Model file for the job. Use its own axes, mm. A direction names the side the tool comes from. Coordinates: 2 decimals unless noted, no trailing zeros. Write each loop counter-clockwise with the first axis right and the second up, starting at its lowest first coordinate (ties: lowest second). Pieces come first, ordered by that corner, then holes. Notation, with made-up numbers: (75.25, -30.75) - (80.25, -30.75) arc R20 cw to (80.25, -0.75) - close; hole circle Ø11 at (14.25, -14.5). An arc over 180 degrees is marked (long way). Put each result on its own line as item: value. Start each with the question number.
1. Saw through at B-B, the plane y = 68. Give the number of separate pieces and of enclosed holes in the cut face, plus the area to 3 significant figures.
2. Saw through at A-A, the plane x = -1. Write the cut outline in (y, z), plus the area to 3 significant figures.
3. Saw through at D-D, the plane z = 2. Write the cut outline in (x, y), plus the area to 3 significant figures.
4. Which spindle directions (+Z, -Z, +X, -X, +Y, -Y) get a long thin tool onto all of the face, cutting with end or side? Do faces 1 (the face through (102, 41, 76.483)), 2 (the face through (-3, 10, 11.5)), 3 (the face through (102, 31, 115.138)). Say none if no direction does.
5. Drill centre lines: L1, parallel to Y at x = 164.5, z = 72; L2, parallel to Y at x = 167, z = 89; L3, parallel to Z at x = 10, y = 12. Where is each one in solid material? Low to high. Write a range as from..to.
6. Drop flat-ended pins along their axis: P1, Ø16.5, axis at x = 91, z = 2.5, coming from the +Y side; P2, Ø1, axis at x = 7, y = 36.5, coming from the -Z side. Give the stop position or say it passes through.
7. Pull direction Z, two halves, no side cores. Call faces 4 (the face through (203, 15, 0)), 5 (the face through (102, 44.52, 79)), 6 (the face through (108, 5, 0)), 7 (the face through (102, 55, 86.614)): released by +Z, released by -Z, zero draft, split by the parting line, or undercut.
8. Saw through at C-C, the plane y = 8. Write the cut outline in (x, z).
```python
from build123d import *

# Parameters (mm, degrees)
SKETCH_1_W            = 100
SKETCH_1_H            = 50
EXTRUDE_1_DEPTH       = 200
SKETCH_2_W            = 192
SKETCH_2_H            = 92
CUT_EXTRUDE_1_DEPTH   = 20
SKETCH_3_W            = 100
SKETCH_3_H            = 50
EXTRUDE_2_DEPTH       = 20
SKETCH_4_W            = 100
SKETCH_4_H            = 50
EXTRUDE_3_DEPTH       = 20
SKETCH_6_W            = 23
SKETCH_6_H            = 10
CUT_EXTRUDE_2_DEPTH   = 15
SKETCH_7_W            = 23
SKETCH_7_H            = 10
CUT_EXTRUDE_3_DEPTH   = 15
SKETCH_10_R           = 21.643075995
SKETCH_10_R_2         = 21.043075995
SKETCH_10_W           = 0.6
SKETCH_10_H           = 92
CUT_EXTRUDE_2_2_DEPTH = 0.05
EXTRUDE_4_DEPTH       = 240
SKETCH_12_W           = 30.390175899
SKETCH_12_H           = 33.741429703
EXTRUDE_5_DEPTH       = 4
SKETCH_13_W           = 30.390175899
SKETCH_13_H           = 33.741429703
EXTRUDE_6_DEPTH       = 4
SKETCH_14_R           = 0.75
EXTRUDE_7_DEPTH       = 27.291157


with BuildPart() as part:
    # 草圖1 → 填料-伸長1 (new body)
    with BuildSketch(Plane(origin=(0, 0, 0), x_dir=(0, 0, -1), z_dir=(1, 0, 0))):
        Rectangle(SKETCH_1_W, SKETCH_1_H)
    extrude(amount=EXTRUDE_1_DEPTH)

    # 草圖2 → 除料-伸長1 (cut)
    with BuildSketch(Plane(origin=(0, 25, 0), x_dir=(1, 0, 0), z_dir=(0, 1, 0))):
        with Locations((100, 0)):
            Rectangle(SKETCH_2_W, SKETCH_2_H)
    extrude(amount=-CUT_EXTRUDE_1_DEPTH, mode=Mode.SUBTRACT)

    # 草圖3 → 填料-伸長2 (add)
    with BuildSketch(Plane.ZY):
        Rectangle(SKETCH_3_W, SKETCH_3_H)
    extrude(amount=EXTRUDE_2_DEPTH)

    # 草圖4 → 填料-伸長3 (add)
    with BuildSketch(Plane(origin=(200, 0, 0), x_dir=(0, 0, -1), z_dir=(1, 0, 0))):
        Rectangle(SKETCH_4_W, SKETCH_4_H)
    extrude(amount=EXTRUDE_3_DEPTH)

    # 草圖6 → Cut-Extrude 2 (cut)
    with BuildSketch(Plane(origin=(4, 0, 0), x_dir=(0, 0, -1), z_dir=(1, 0, 0))):
        with Locations((0, 10)):
            Rectangle(SKETCH_6_W, SKETCH_6_H)
    extrude(amount=-CUT_EXTRUDE_2_DEPTH, mode=Mode.SUBTRACT)

    # 草圖7 → 除料-伸長3 (cut)
    with BuildSketch(Plane.ZY.offset(-196)):
        with Locations((0, 10)):
            Rectangle(SKETCH_7_W, SKETCH_7_H)
    extrude(amount=-CUT_EXTRUDE_3_DEPTH, mode=Mode.SUBTRACT)

    # 草圖10 → Cut-Extrude 2 2 (cut)
    with BuildSketch(Plane(origin=(0, 5, 0), x_dir=(1, 0, 0), z_dir=(0, 1, 0))):
        with Locations((100, 0)):
            Circle(SKETCH_10_R)
        with Locations((100, 0)):
            Circle(SKETCH_10_R_2, mode=Mode.SUBTRACT)
        with Locations((100, 0)):
            Rectangle(SKETCH_10_W, SKETCH_10_H)
    extrude(amount=-CUT_EXTRUDE_2_2_DEPTH, mode=Mode.SUBTRACT)

    # 草圖11 → 填料-伸長4 (add)
    with BuildSketch(Plane(origin=(220, 0, 0), x_dir=(0, 0, -1), z_dir=(1, 0, 0))):
        Polygon((-50, 25), (-56.223345598, 25), (-56.223345598, 33.611091941), (-59.145477896, 33.611091941), (-59.145477896, 27.182400885), (-64.794933673, 27.182400885), (-64.794933673, 32.052621382), (-70.054771809, 32.052621382), (-70.054771809, 38.481312437), (-76.483462864, 38.481312437), (-76.483462864, 44.520385853), (-81.938109821, 44.520385853), (-81.938109821, 50.949076909), (-86.613521497, 50.949076909), (-86.613521497, 58.741429703), (-107.458065223, 58.741429703), (-107.458065223, 80.646512644), (-50, 80.646512644), (-50, 86.032586896), (-115.138208137, 86.032586896), (-115.138208137, -25), (-50, -25), align=None)
    extrude(amount=-EXTRUDE_4_DEPTH)

    # 草圖12 → 填料-伸長5 (add)
    with BuildSketch(Plane(origin=(220, 0, 0), x_dir=(0, 0, -1), z_dir=(1, 0, 0))):
        with Locations((-71.418433548, 41.870714851)):
            Rectangle(SKETCH_12_W, SKETCH_12_H)
    extrude(amount=-EXTRUDE_5_DEPTH)

    # 草圖13 → 填料-伸長6 (add)
    with BuildSketch(Plane.ZY.offset(20)):
        with Locations((71.418433548, 41.870714851)):
            Rectangle(SKETCH_13_W, SKETCH_13_H)
    extrude(amount=-EXTRUDE_6_DEPTH)

    # 草圖14 → 填料-伸長7 (add)
    with BuildSketch(Plane(origin=(0, 86.032586896, 0), x_dir=(1, 0, 0), z_dir=(0, 1, 0))):
        with Locations((218.161156155, -76.375011751)):
            Circle(SKETCH_14_R)
        with Locations((218.161156155, -73.375011751)):
            Circle(SKETCH_14_R)
        with Locations((218.161156155, -70.375011751)):
            Circle(SKETCH_14_R)
        with Locations((218.161156155, -67.375011751)):
            Circle(SKETCH_14_R)
        with Locations((218.161156155, -64.375011751)):
            Circle(SKETCH_14_R)
        with Locations((218.161156155, -61.375011751)):
            Circle(SKETCH_14_R)
        with Locations((218.161156155, -58.375011751)):
            Circle(SKETCH_14_R)
        with Locations((-18.761156155, -85.375011751)):
            Circle(SKETCH_14_R)
        with Locations((-18.761156155, -79.375011751)):
            Circle(SKETCH_14_R)
        with Locations((-18.761156155, -70.375011751)):
            Circle(SKETCH_14_R)
        with Locations((218.161156155, -85.375011751)):
            Circle(SKETCH_14_R)
        with Locations((218.161156155, -82.375011751)):
            Circle(SKETCH_14_R)
        with Locations((218.161156155, -79.375011751)):
            Circle(SKETCH_14_R)
        with Locations((-18.761156155, -82.375011751)):
            Circle(SKETCH_14_R)
        with Locations((-18.761156155, -76.375011751)):
            Circle(SKETCH_14_R)
        with Locations((-18.761156155, -73.375011751)):
            Circle(SKETCH_14_R)
        with Locations((-18.761156155, -67.375011751)):
            Circle(SKETCH_14_R)
        with Locations((-18.761156155, -64.375011751)):
            Circle(SKETCH_14_R)
    extrude(amount=-EXTRUDE_7_DEPTH)


solid = part.part
```
Final values:
1. separate pieces: 19
1. enclosed holes: 0
1. area: 1,880 mm²
2. outline: (-25, -50) - (25, -50) - (25, 56.22) - (33.61, 56.22) - (33.61, 59.15) - (27.18, 59.15) - (27.18, 64.79) - (32.05, 64.79) - (32.05, 70.05) - (38.48, 70.05) - (38.48, 76.48) - (44.52, 76.48) - (44.52, 81.94) - (50.95, 81.94) - (50.95, 86.61) - (58.74, 86.61) - (58.74, 107.46) - (80.65, 107.46) - (80.65, 50) - (86.03, 50) - (86.03, 115.14) - (-25, 115.14) - close; hole (5, -11.5) - (15, -11.5) - (15, 11.5) - (5, 11.5) - close
2. area: 9,900 mm²
3. outline: (-20, -25) - (220, -25) - (220, 25) - (196, 25) - (196, 15) - (211, 15) - (211, 5) - (121.55, 5) - (121.55, 4.95) - (120.95, 4.95) - (120.95, 5) - (100.3, 5) - (100.3, 4.95) - (99.7, 4.95) - (99.7, 5) - (79.05, 5) - (79.05, 4.95) - (78.45, 4.95) - (78.45, 5) - (-11, 5) - (-11, 15) - (4, 15) - (4, 25) - (-20, 25) - close
3. area: 7,860 mm²
4. face 1: -Z
4. face 2: none
4. face 3: +Z, +X, -X, +Y, -Y
5. L1: y = -25..38.48, 80.65..86.03
5. L2: y = -25..58.74, 80.65..86.03
5. L3: z = -50..-46, 46..115.14
6. P1: stops at y = 5
6. P2: stops at z = 70.05
7. face 4: undercut
7. face 5: zero draft
7. face 6: undercut
7. face 7: released by -Z
8. outline: (-20, -50) - (220, -50) - (220, 115.14) - (-20, 115.14) - close; hole (-11, -11.5) - (4, -11.5) - (4, -46) - (196, -46) - (196, -11.5) - (211, -11.5) - (211, 11.5) - (196, 11.5) - (196, 46) - (4, 46) - (4, 11.5) - (-11, 11.5) - close
